from build123d import *

# Parameters (mm, degrees)
SKETCH1_W           = 45
SKETCH1_H           = 45
SKETCH1_R           = 3.5
BOSS_EXTRUDE1_DEPTH = 2.032
FILLET2_R           = 5
SKETCH4_R           = 1.6
CUT_EXTRUDE3_DEPTH  = 3.032
SKETCH5_W           = 3
SKETCH5_H           = 1.5
CUT_EXTRUDE5_DEPTH  = 3.032


with BuildPart() as part:
    # Sketch1 → Boss-Extrude1 (new body)
    with BuildSketch(Plane.XY):
        with Locations((16.5, 0)):
            Rectangle(SKETCH1_W, SKETCH1_H)
        Circle(SKETCH1_R, mode=Mode.SUBTRACT)
    extrude(amount=BOSS_EXTRUDE1_DEPTH)

    # Fillet2
    fillet2_edges = [part.edges().sort_by_distance(p)[0] for p in [
        (39, -22.5, 1.016),
        (-6, -22.5, 1.016),
        (-6, 22.5, 1.016),
        (39, 22.5, 1.016),
    ]]
    fillet(fillet2_edges, radius=FILLET2_R)

    # Sketch4 → Cut-Extrude3 (cut, through all)
    with BuildSketch(Plane(origin=(0, 0, 0), x_dir=(-1, 0, 0), z_dir=(0, 0, -1))):
        with Locations((-31.5, 15)):
            Circle(SKETCH4_R)
        with Locations((-31.5, 0)):
            Circle(SKETCH4_R)
        with Locations((-31.5, -15)):
            Circle(SKETCH4_R)
    extrude(amount=-CUT_EXTRUDE3_DEPTH, mode=Mode.SUBTRACT)

    # Sketch5 → Cut-Extrude5 (cut, through all)
    with BuildSketch(Plane(origin=(0, 0, 0), x_dir=(-1, 0, 0), z_dir=(0, 0, -1))):
        with Locations((0, 8.25)):
            Rectangle(SKETCH5_W, SKETCH5_H)
        with Locations((0, -8.25)):
            Rectangle(SKETCH5_W, SKETCH5_H)
    extrude(amount=-CUT_EXTRUDE5_DEPTH, mode=Mode.SUBTRACT)


solid = part.part
The listing builds one solid part. Answer for the finished solid, in the listing's coordinates (mm). A direction names the side the tool comes from. Coordinates: 2 decimals unless noted, no trailing zeros. Loops run counter-clockwise (first coordinate to the right, second up) from the corner with the lowest first, then second, coordinate; pieces in that order, holes last. Notation, with made-up numbers: (-8, 81.5) -> (-3, 81.5) arc R6 cw to (-3, 87.5) -> close; hole circle Ø1 at (37, 50.5). An arc over 180 degrees is marked (long way). Write item = value, one per line. Start each with the question number.
1) The mould has two halves that part along Y. Classify faces 1 (the face through (39, 0, 1)), 2 (the face through (0, -7.5, 1)), 3 (the face through (-4.57, 21, 1.03)), 4 (the face through (37.5, -21.07, 1.03)): released by +Y, released by -Y, zero draft, split by the parting line, or undercut.
2) Given pin 1 Ø2.5 at (x, y) = (31.5, -15) entering from +Z, flat-ended and moving along its own axis, determine where the tip first touches the part or whether it passes through.
3) A cutting plane is placed at D-D (z = 0.75). Give the vertices of the cut face in (x, y), then the cut area to 3 significant figures.
4) A tool of negligible diameter and unlimited length cuts with its end or side. For faces 5 (the face through (0, -9, 1)), 6 (the face through (-4.57, -21, 1.03)), from which of +Z, -Z, +X, -X, +Y, -Y can it reach the whole face along a straight path? Write none if from no direction.
5) A cutting plane is placed at B-B (x = 31.5). Give the vertices of the cut face in (y, z).
6) A cutting plane is placed at C-C (y = 15). Give the vertices of the cut face in (x, z).
7) Straight lines are drawn through the part: line 1 (Y direction, x = 31.5, z = 1.05); line 2 (Y direction, x = 0, z = 0.8); line 3 (Y direction, x = -3, z = 0.5). For each, find the intervals that lie inside material, in ascending order. Write a range as from..to.
8) A cutting plane is placed at A-A (y = 0). Give the vertices of the cut face in (x, z), then the cut area to 3 significant figures.
Responses:
q1.face_1 = zero draft
q1.face_2 = undercut
q1.face_3 = released by +Y
q1.face_4 = released by -Y
q2.pin_1 = through
q3.outline = (-6, -17.5) arc R5 ccw to (-1, -22.5) -> (34, -22.5) arc R5 ccw to (39, -17.5) -> (39, 17.5) arc R5 ccw to (34, 22.5) -> (-1, 22.5) arc R5 ccw to (-6, 17.5) -> close; hole circle Ø7 at (0, 0); hole (-1.5, -9) -> (1.5, -9) -> (1.5, -7.5) -> (-1.5, -7.5) -> close; hole (-1.5, 7.5) -> (1.5, 7.5) -> (1.5, 9) -> (-1.5, 9) -> close; hole circle Ø3.2 at (31.5, -15); hole circle Ø3.2 at (31.5, 0); hole circle Ø3.2 at (31.5, 15)
q3.area = 1,930 mm²
q4.face_5 = +Z, -Z
q4.face_6 = +Z, -Z, -X, -Y
q5.outline = (-22.5, 0) -> (-16.6, 0) -> (-16.6, 2.03) -> (-22.5, 2.03) -> close; (-13.4, 0) -> (-1.6, 0) -> (-1.6, 2.03) -> (-13.4, 2.03) -> close; (1.6, 0) -> (13.4, 0) -> (13.4, 2.03) -> (1.6, 2.03) -> close; (16.6, 0) -> (22.5, 0) -> (22.5, 2.03) -> (16.6, 2.03) -> close
q6.outline = (-6, 0) -> (29.9, 0) -> (29.9, 2.03) -> (-6, 2.03) -> close; (33.1, 0) -> (39, 0) -> (39, 2.03) -> (33.1, 2.03) -> close
q7.line_1 = -22.5..-16.6, -13.4..-1.6, 1.6..13.4, 16.6..22.5
q7.line_2 = -22.5..-9, -7.5..-3.5, 3.5..7.5, 9..22.5
q7.line_3 = -22.08..-1.8, 1.8..22.08
q8.outline = (-6, 0) -> (-3.5, 0) -> (-3.5, 2.03) -> (-6, 2.03) -> close; (3.5, 0) -> (29.9, 0) -> (29.9, 2.03) -> (3.5, 2.03) -> close; (33.1, 0) -> (39, 0) -> (39, 2.03) -> (33.1, 2.03) -> close
q8.area = 70.7 mm²
